Verification items for this drawing (mm, ordinates from the low corner). A direction names the side the tool comes from. Round coordinates to 2 decimals unless told otherwise and drop trailing zeros. Order: outer loops, then holes, each group sorted by start corner. A loop starts at its lowest first (then second) coordinate and runs counter-clockwise, first axis right, second up. Notation, with made-up numbers: (41, -26) - (79, -26) arc R19 cw to (79, -9) - close; hole circle Ø11 at (63.5, -26). An arc over 180 degrees is marked (long way). Return JSON: item names as keys, results as strings. Group by question number.
Q1. Tool access check on the marked faces 1, 2 and 3. Record the directions out of +Z, -Z, +X, -X, +Y, -Y that give a thin tool (end or side, any length) a straight path to the whole face; none if there is none.
Q2. Gauge pin test, flat ends, axial feed: pin 1 Ø5 at (x, y) = (55, 12.5) entering from -Z; pin 2 Ø3 at (x, y) = (6.5, 5) entering from +Z; pin 3 Ø12 at (x, z) = (33, 16) entering from +Y; pin 4 Ø5 at (x, y) = (33, 29) entering from -Z. Record the tip position at first contact, or that the pin passes through.
Q3. Draft check along Y on the marked faces 4, 5, 6 and 7. Enter one of: pulls with the +Y half, pulls with the -Y half, needs draft (parallel to the pull), parting line crosses it, or undercut.
Q4. Sectioned sample at D-D, the plane z = 15.75. Record the cut outline in (x, y), then the cut area to 3 significant figures.
Q5. Material ranges on line 1 along Y through (x, z) = (57, 22.25); line 2 along Y through (x, z) = (57, 3.4); line 3 along X through (y, z) = (53, 8.25), recorded low to high.
Q6. Sectioned sample at C-C, the plane y = 39.5. Record the cut outline in (x, z), then the cut area to 3 significant figures.
Q7. Sectioned sample at B-B, the plane y = 5.5. Record the cut outline in (x, z), then the cut area to 3 significant figures.
Q8. Sectioned sample at A-A, the plane z = 20. Record the cut outline in (x, y), then the cut area to 3 significant figures.
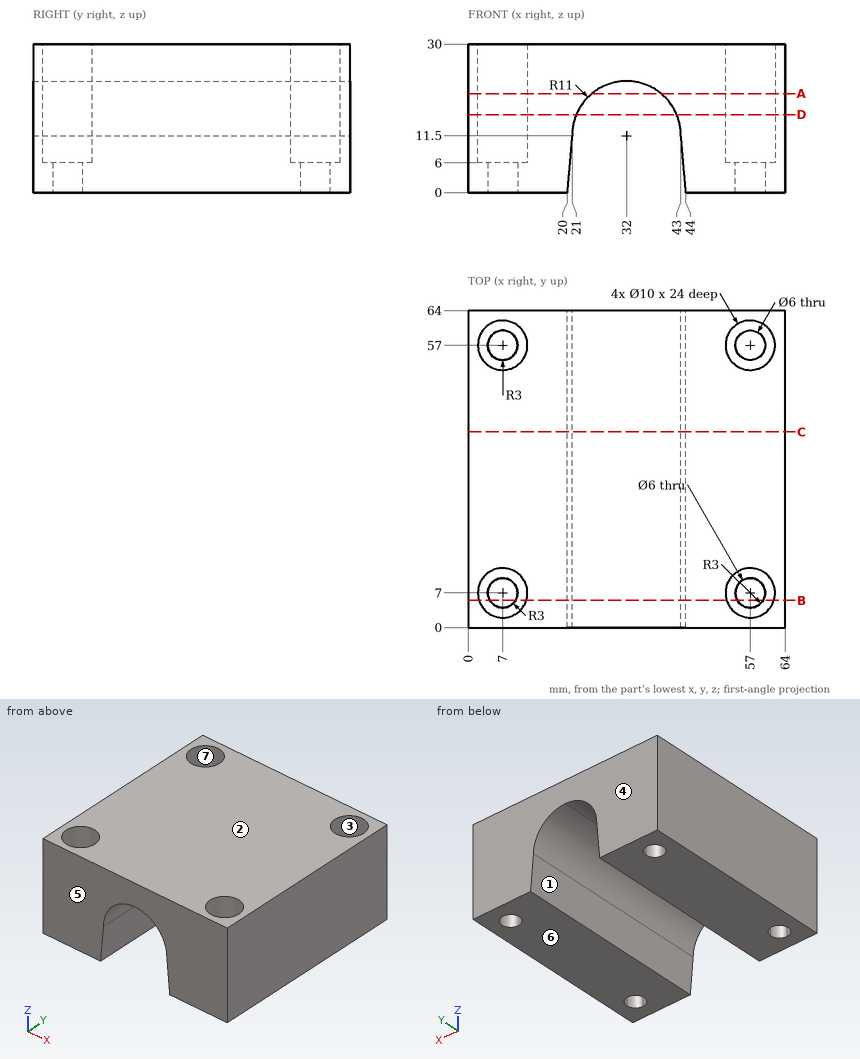
Reply:
{
 "1": {"face 1": "-Z, +Y, -Y", "face 2": "+Z, +X, -X, +Y, -Y", "face 3": "+Z"},
 "2": {"pin 1": "z = 0", "pin 2": "z = 6", "pin 3": "through", "pin 4": "z = 21.93"},
 "3": {"face 4": "pulls with the +Y half", "face 5": "pulls with the -Y half", "face 6": "needs draft", "face 7": "undercut"},
 "4": {"outline": "(0, 0) - (21.85, 0) - (21.85, 64) - (0, 64) - close; (42.15, 0) - (64, 0) - (64, 64) - (42.15, 64) - close; hole circle Ø10 at (7, 7); hole circle Ø10 at (7, 57); hole circle Ø10 at (57, 7); hole circle Ø10 at (57, 57)", "area": "2,480 mm^2"},
 "5": {"line 1": "0 to 2, 12 to 52, 62 to 64", "line 2": "0 to 4, 10 to 54, 60 to 64", "line 3": "0 to 4, 10 to 20.72, 43.28 to 54, 60 to 64"},
 "6": {"outline": "(0, 0) - (20, 0) - (21, 11.5) arc R11 cw to (43, 11.5) - (44, 0) - (64, 0) - (64, 30) - (0, 30) - close", "area": "1,470 mm^2"},
 "7": {"outline": "(0, 0) - (4.4, 0) - (4.4, 6) - (2.23, 6) - (2.23, 30) - (0, 30) - close; (9.6, 0) - (20, 0) - (21, 11.5) arc R11 cw to (43, 11.5) - (44, 0) - (54.4, 0) - (54.4, 6) - (52.23, 6) - (52.23, 30) - (11.77, 30) - (11.77, 6) - (9.6, 6) - close; (59.6, 0) - (64, 0) - (64, 30) - (61.77, 30) - (61.77, 6) - (59.6, 6) - close", "area": "945 mm^2"},
 "8": {"outline": "(0, 0) - (25.02, 0) - (25.02, 64) - (0, 64) - close; (38.98, 0) - (64, 0) - (64, 64) - (38.98, 64) - close; hole circle Ø10 at (7, 7); hole circle Ø10 at (7, 57); hole circle Ø10 at (57, 7); hole circle Ø10 at (57, 57)", "area": "2,890 mm^2"}
}
